```python
from build123d import *

# Parameters (mm, degrees)
SKETCH1_R          = 406.4
EXTRUDE1_DEPTH     = 30
SKETCH2_R          = 17.526
CUT_EXTRUDE1_DEPTH = 31
CIRPATTERN1_COUNT  = 20


with BuildPart() as part:
    # Sketch1 → Extrude1 (new body)
    with BuildSketch(Plane.XY):
        Circle(SKETCH1_R)
    extrude(amount=EXTRUDE1_DEPTH)

    # Sketch2 → Cut-Extrude1 (cut, through all)
    with BuildSketch(Plane(origin=(0, 0, 0), x_dir=(-1, 0, 0), z_dir=(0, 0, -1))):
        with Locations((58.608172327, 370.037436804)):
            Circle(SKETCH2_R)
    cut_extrude1 = extrude(amount=-CUT_EXTRUDE1_DEPTH, mode=Mode.SUBTRACT)

    # CirPattern1: Cut-Extrude1 ×20 about axis
    cirpattern1_axis = Axis((0, 0, 0), (0, 0, 1))
    for i in range(1, CIRPATTERN1_COUNT):
        add(cut_extrude1.rotate(cirpattern1_axis, i * 360 / CIRPATTERN1_COUNT), mode=Mode.SUBTRACT)


solid = part.part
```
The listing builds one solid part. Answer for the finished solid, in the listing's coordinates (mm). Give positions to 0.01 mm unless a question says otherwise; leave off trailing zeros. Write each loop counter-clockwise with the first axis right and the second up, starting at its lowest first coordinate (ties: lowest second). Pieces come first, ordered by that corner, then holes. Notation, with made-up numbers: (43.5, 65) - (82.5, 65) arc R36 ccw to (82.5, 100) - close; hole circle Ø1 at (-30, -4.75). An arc over 180 degrees is marked (long way). Use one line per item in the form item = value. Start each with the question number.
1) Consider line 1 along Y through (x, z) = (-274, 13.5); line 2 along X through (y, z) = (339, 18.25); line 3 along X through (y, z) = (-343, 18.25). Determine where each line is inside the solid, lowest interval first. Write a range as from..to.
2) Flat-ended cylindrical pins translate along their axes: pin 1 Ø2 at (y, z) = (37, 4) entering from -X; pin 2 Ø12 at (x, z) = (-71.5, 26.5) entering from -Y; pin 3 Ø1 at (x, z) = (305, 9.5) entering from +Y. Find the tip coordinate at first contact, or state that the pin passes through.
3) Find section B-B on x = -140. Determine the outline of the cut face in (y, z).
4) Find section A-A on z = 20.75. Count the separate pieces of the cut face and the enclosed holes in it, plus the area to 3 significant figures.
5) The mould has two halves that part along X. Classify faces 1 (the face through (-88.1, -396.736, 14.79)), 2 (the face through (-6, 6, 0)), 3 (the face through (387.414, 56.327, 14.79)): pulls with the +X half, pulls with the -X half, needs draft (parallel to the pull), parting line crosses it, or undercut.
6) Find section C-C on y = 292. Determine the outline of the cut face in (x, z), plus the area to 3 significant figures.
Geometry results:
q1.line_1 = -300.14..-279.91, -249.93..249.93, 279.91..300.14
q1.line_2 = -224.14..-186.83, -153.35..153.35, 186.83..224.14
q1.line_3 = -217.97..-185.01, -155.16..155.16, 185.01..217.97
q2.pin_1 = -404.8
q2.pin_2 = -401.09
q2.pin_3 = 269.15
q3.outline = (-381.52, 0) - (381.52, 0) - (381.52, 30) - (-381.52, 30) - close
q4.separate_pieces = 1
q4.enclosed_holes = 20
q4.area = 500,000 mm2
q5.face_1 = parting line crosses it
q5.face_2 = needs draft
q5.face_3 = undercut
q6.outline = (-282.66, 0) - (282.66, 0) - (282.66, 30) - (-282.66, 30) - close
q6.area = 17,000 mm2
